from build123d import *

# Parameters (mm, degrees)
F1_DEPTH = 3.175
F3_DEPTH = 3.175


with BuildPart() as f1:
    # F0 (on Front) → F1 (new body)
    with BuildSketch(Plane.XZ):
        with BuildLine():
            Line((50.8, -73.025), (50.8, 73.025))
            ThreePointArc((50.8, 73.025), (44.290448, 88.740448), (28.575, 95.25))
            Line((28.575, 95.25), (-28.575, 95.25))
            ThreePointArc((-28.575, 95.25), (-44.290448, 88.740448), (-50.8, 73.025))
            Line((-50.8, 73.025), (-50.8, -73.025))
            ThreePointArc((-50.8, -73.025), (-44.290448, -88.740448), (-28.575, -95.25))
            Line((-28.575, -95.25), (28.575, -95.25))
            ThreePointArc((28.575, -95.25), (44.290448, -88.740448), (50.8, -73.025))
        make_face()
    extrude(amount=F1_DEPTH)

    # F2 (on face) → F3 (join)
    with BuildSketch(Plane.XZ.offset(3.175)):
        with BuildLine():
            Line((-53.975, 73.025), (-53.975, -73.025))
            ThreePointArc((-53.975, -73.025), (-46.535512, -90.985512), (-28.575, -98.425))
            Line((-28.575, -98.425), (28.575, -98.425))
            ThreePointArc((28.575, -98.425), (46.535512, -90.985512), (53.975, -73.025))
            Line((53.975, -73.025), (53.975, 73.025))
            ThreePointArc((53.975, 73.025), (46.535512, 90.985512), (28.575, 98.425))
            Line((28.575, 98.425), (-28.575, 98.425))
            ThreePointArc((-28.575, 98.425), (-46.535512, 90.985512), (-53.975, 73.025))
        make_face()
    extrude(amount=F3_DEPTH)


solid = f1.part
For this review, take the finished solid that the model builds, in its own axes (mm). A direction names the side the tool comes from. Round coordinates to 2 decimals unless told otherwise and drop trailing zeros. Write each loop counter-clockwise with the first axis right and the second up, starting at its lowest first coordinate (ties: lowest second). Pieces come first, ordered by that corner, then holes. Notation, with made-up numbers: (-21, 53.5) -> (-1, 53.5) arc R7 cw to (-1, 59.5) -> close; hole circle Ø7 at (82, 0.25). An arc over 180 degrees is marked (long way). Use CSV: the item, a comma, the result in double quotes.
(1) To check wall thickness, follow L1, parallel to Z at x = -2, y = -0.75; L2, parallel to X at y = -1.75, z = -37; L3, parallel to X at y = -3, z = 90. State the ranges of each line that lie inside material, in increasing order. Write a range as [from, to].
Computed values:
L1,"[-95.25, 95.25]"
L2,"[-50.8, 50.8]"
L3,"[-42.92, 42.92]"
(2) For faces 1 (the face through (44.46, -1.57, 88.57)), 2 (the face through (-44.12, -1.57, 88.91)), 3 (the face through (-44.46, -1.57, -88.57)), 4 (the face through (44.12, -1.57, -88.91)), list the 3-axis set-ups (+Z, -Z, +X, -X, +Y, -Y) from which the entire face can be reached by the end or side of a thin tool; tool diameter is ignored.
Computed values:
face 1,"+Z, +X, +Y"
face 2,"+Z, -X, +Y"
face 3,"-Z, -X, +Y"
face 4,"-Z, +X, +Y"
(3) Clearance check with flat-ended pins moving along their axes: P1, Ø1.5, axis at x = -36.5, y = -2.5, coming from the +Z side; P2, Ø1, axis at x = -11.5, y = -2, coming from the +Z side; P3, Ø1, axis at y = -1, z = -7, coming from the +X side. State where each tip first meets the part, or that it passes through.
Computed values:
P1,"z = 97.26"
P2,"z = 95.25"
P3,"x = 50.8"
(4) Consider section A-A, the plane z = -57. Give the boundary of the cut face in (x, y) (3 decimals).
Computed values:
outline,"(-53.975, -6.35) -> (53.975, -6.35) -> (53.975, -3.175) -> (50.8, -3.175) -> (50.8, 0) -> (-50.8, 0) -> (-50.8, -3.175) -> (-53.975, -3.175) -> close"
(5) Consider section B-B, the plane y = -1.25. Give the boundary of the cut face in (x, z) (3 decimals), plus the area to 3 significant figures.
Computed values:
outline,"(-50.8, -73.025) arc R22.225 ccw to (-28.575, -95.25) -> (28.575, -95.25) arc R22.225 ccw to (50.8, -73.025) -> (50.8, 73.025) arc R22.225 ccw to (28.575, 95.25) -> (-28.575, 95.25) arc R22.225 ccw to (-50.8, 73.025) -> close"
area,"18,900 mm²"
